Autodesk Inventor part; units mm, degrees
ref_plane "YZ Plane" through (0, 0, 0) normal (1, 0, 0) x (0, 1, 0)
ref_plane "XY Plane" through (0, 0, 0) normal (0, 0, 1) x (1, 0, 0)
sketch "Sketch1" plane through (0, 0, 0) normal (0, 0, 1) x (1, 0, 0)
  line L0 (-135.8451, 94.4022) -> (-5.8451, 19.3467)
  line L1 (-134.5951, 96.5673) -> (-4.5951, 21.5118)
  line L2 (-4.5951, 21.5118) -> (-5.8451, 19.3467)
  line L3 (-134.5951, 96.5673) -> (-135.8451, 94.4022)
  line L4 (-164.6473, 0) -> (36.9683, 0)
  point P0 (0, 0)
  dimension "d0" = 2.5
  dimension "d3" = 130
  dimension "d4" = 30
extrude "Extrusion1" add sketch "Sketch1" along normal blind 67
sketch "Sketch2" plane through (-134.5951, 96.5673, 67) normal (0.5, 0.866, 0) x (0.866, -0.5, 0)
  point P0 (164.8464, 67)
sketch "Sketch4" plane through (0, 0, 67) normal (0, 0, 1) x (1, 0, 0)
  point P0 (0, 0)
sketch "Sketch5" plane through (-134.5951, 96.5673, 67) normal (0.5, 0.866, 0) x (0.866, -0.5, 0)
  line L0 (0, 67) -> (0, 0)
  line L1 (0, 0) -> (152, 0)
  line L2 (152, 0) -> (152, 4)
  line L3 (152, 4) -> (0, 4)
  line L4 (0, 4) -> (0, 0)
  point P0 (164.8464, 67)
  point P1 (0, 4)
sketch "Sketch6" plane through (-134.5951, 96.5673, 67) normal (0.5, 0.866, 0) x (0.866, -0.5, 0)
  line L0 (0, 67) -> (150.1111, 67)
  line L1 (0, 67) -> (150.1111, 67)
  line L2 (150.1111, 67) -> (150.1111, 62)
  line L3 (150.1111, 62) -> (0, 62)
  line L4 (0, 62) -> (0, 67)
  point P0 (164.8464, 67)
extrude "Extrusion2" add sketch "Sketch5" along normal blind 43
extrude "Extrusion3" add sketch "Sketch6" along normal blind 43
ref_plane "Work Plane1" through (0, 19.347, 0) normal (0, 1, 0) x (-1, 0, 0)
sketch "Sketch8" plane through (0, 19.347, 0) normal (0, 1, 0) x (-1, 0, 0)
  line L0 (5.8451, 67) -> (4.5951, 67)
  line L1 (4.5951, 67) -> (-90.4049, 67)
  line L2 (-90.4049, 67) -> (-90.4049, 0)
  line L3 (-90.4049, 0) -> (4.5951, 0)
  line L4 (4.5951, 0) -> (4.5951, 67)
  point P0 (0, 0)
  dimension "d10" = 95
extrude "Extrusion4" add sketch "Sketch8" along normal blind 43
sketch "Sketch9" plane through (0, 62.347, 0) normal (0, 1, 0) x (1, 0, 0)
  line L0 (-113.0951, -5) -> (10.6762, -5)
  line L1 (0, -5) -> (86, -5)
  line L2 (86, -5) -> (86, -63)
  line L3 (86, -63) -> (0, -63)
  line L4 (0, -63) -> (0, -5)
  point P0 (0, 0)
extrude "Extrusion5" cut sketch "Sketch9" against normal through all
sketch "Sketch12" plane through (0, 62.347, 63) normal (1, 0, 0) x (0, 0, -1)
  line L0 (-4, 0) -> (0, 0)
  line L1 (58, 0) -> (58, -43)
  line L2 (0, 0) -> (58, 0)
  line L3 (58, 0) -> (58, -40)
  line L4 (58, -40) -> (0, -40)
  line L5 (0, -40) -> (0, 0)
  point P0 (63, -62.347)
extrude "Extrusion6" cut sketch "Sketch12" against normal blind 10
properties part number "channel"
Could you check a few things on this model? Use its own coordinates, in mm. A direction names the side the tool comes from. Round coordinates to 2 decimals unless told otherwise and drop trailing zeros. Loops run counter-clockwise (first coordinate to the right, second up) from the corner with the lowest first, then second, coordinate; pieces in that order, holes last. Notation, with made-up numbers: M 32,53.5 L 57,53.5 A16 cw 57,84.5 Z; hole C 13,-36 d4. An arc over 180 degrees is marked long. Write item = value, one per line.
1. I want a section at A-A, the plane x = 64.5. Write out the boundary of the cut face in (y, z), and give its area (3 significant figures).
Results below:
outline = M 19.35,0 L 62.35,0 L 62.35,5 L 19.35,5 Z; M 19.35,63 L 62.35,63 L 62.35,67 L 19.35,67 Z
area = 387 mm²
2. Which directions (+Z, -Z, +X, -X, +Y, -Y) give clear straight access to the entire face, cutting with the end or side of a thin tool? Please do faces 1 (the face through (-73.17, 61.103, 33.594)), 2 (the face through (86, 41, 34)), 3 (the face through (86.2, 62.347, 31.2)).
Results below:
face_1 = +Y
face_2 = +Y, -Y
face_3 = +Z, -Z, +X, +Y
3. I need wall thicknesses on probe 1 along Z at (x, y) = (9, 49.5); probe 2 along X at (y, z) = (45, 54); probe 3 along X at (y, z) = (35.5, 40). Which ranges of each line are inside material? Lowest first, please.
Results below:
probe_1 = 0 to 5, 63 to 67
probe_2 = -50.28 to -45.28, 86 to 90.4
probe_3 = -33.82 to -28.82, 86 to 90.4
4. I want a section at C-C, the plane y = 36.5. Write out the boundary of the cut face in (x, z).
Results below:
outline = M -35.56,0 L 90.4,0 L 90.4,67 L -35.56,67 Z; hole M -30.56,5 L 86,5 L 86,63 L -30.56,63 Z
5. Will these pins go through, and if not, where does the flat tip stop? P1, Ø1.2, axis at x = -8.5, z = 23, coming from the +Y side; P2, Ø6, axis at x = 42, z = 7.5, coming from the +Y side; P3, Ø2, axis at y = 97, z = 45, coming from the -X side.
Results below:
P1 = 22.35
P2 = 62.35
P3 = -134.92
6. I want a section at B-B, the plane y = 116. Write out the boundary of the cut face in (x, z).
Results below:
outline = M -123.38,0 L -82.25,0 L -82.25,5 L -123.38,5 Z; M -123.38,63 L -82.25,63 L -82.25,67 L -123.38,67 Z
